Could you check a few things on this model? Use its own coordinates, in mm. Face numbers are marked on the shaded views. A direction names the side the tool comes from. Give positions to 0.01 mm unless a question says otherwise; leave off trailing zeros. Order: outer loops, then holes, each group sorted by start corner. A loop starts at its lowest first (then second) coordinate and runs counter-clockwise, first axis right, second up. Notation, with made-up numbers: M -34.5,12.5 L 5.5,12.5 A32 ccw 5.5,39.5 Z; hole C 3.5,16 d1. An arc over 180 degrees is marked long. Answer in a Markdown table with one row per item. Add a question column.
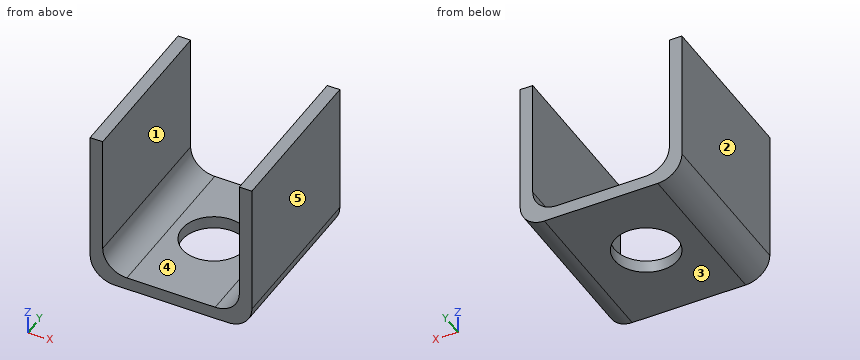
```python
from build123d import *

# Parameters (mm, degrees)
BOSS_EXTRUDE1_DEPTH = 8.636
HOLE1_D             = 3.3274


with BuildPart() as part:
    # Sketch1 → Boss-Extrude1 (new body)
    with BuildSketch(Plane(origin=(0, 11.385459202, 0), x_dir=(-1, 0, 0), z_dir=(0, 1, 0))):
        with BuildLine():
            Line((5.749291724, 0), (11.718291724, 0))
            ThreePointArc((11.718291724, 0), (12.616317336, 0.371974388), (12.988291724, 1.27))
            Line((12.988291724, 1.27), (12.988291724, 8.2296))
            Line((12.988291724, 8.2296), (12.327891724, 8.2296))
            Line((12.327891724, 8.2296), (12.327891724, 1.9304))
            ThreePointArc((12.327891724, 1.9304), (11.955917336, 1.032374388), (11.057891724, 0.6604))
            Line((11.057891724, 0.6604), (6.409691724, 0.6604))
            ThreePointArc((6.409691724, 0.6604), (5.511666112, 1.032374388), (5.139691724, 1.9304))
            Line((5.139691724, 1.9304), (5.139691724, 8.2296))
            Line((5.139691724, 8.2296), (4.479291724, 8.2296))
            Line((4.479291724, 8.2296), (4.479291724, 1.27))
            ThreePointArc((4.479291724, 1.27), (4.851266112, 0.371974388), (5.749291724, 0))
        make_face()
    extrude(amount=-BOSS_EXTRUDE1_DEPTH)

    # Hole1 (through all)
    with Locations(Plane.XY.offset(0.6604)):
        with Locations((-8.886505488, 7.234194178)):
            Hole(HOLE1_D / 2)


solid = part.part
```
1. Suppose I cut it at D-D on x = -6. List the corners of the cut face in (y, z) for me, plus the area to 3 significant figures.
2. Will this pin go through, and if not, where does the flat tip stop? P1, Ø2.5, axis at x = -9, y = 5, coming from the +Z side.
3. If I drill on line 1 along X through (y, z) = (10.75, 2); line 2 along Z through (x, y) = (-10.5, 10); line 3 along X through (y, z) = (5.75, 1.75), over which ranges is the centre line in solid material (lowest first)? Write a range as [from, to].
4. Suppose I cut it at B-B on y = 4. List the corners of the cut face in (x, z) for me.
5. Thinking about a two-plate mould opening in X: for the marked faces 3, 4 and 5, which applies, pulls with the +X half, pulls with the -X half, needs draft (parallel to the pull), parting line crosses it, or undercut?
6. Suppose I cut it at A-A on z = 4.75. List the corners of the cut face in (x, y) for me.
7. Suppose I cut it at C-C on y = 8. List the corners of the cut face in (x, z) for me, plus the area to 3 significant figures.
8. For the marked faces 1 and 2, which set-ups out of +Z, -Z, +X, -X, +Y, -Y let a thin tool reach every point of the face, with its end or its side?
Findings below:
| question | item | result |
|---|---|---|
| 1 | outline | M 2.75,0 L 11.39,0 L 11.39,0.73 L 2.75,0.73 Z |
| 1 | area | 6.29 mm2 |
| 2 | P1 | z = 0.66 |
| 3 | line 1 | [-12.99, -12.33], [-5.14, -4.48] |
| 3 | line 2 | [0, 0.66] |
| 3 | line 3 | [-12.99, -12.32], [-5.15, -4.48] |
| 4 | outline | M -12.99,1.27 A1.27 ccw -11.72,0 L -5.75,0 A1.27 ccw -4.48,1.27 L -4.48,8.23 L -5.14,8.23 L -5.14,1.93 A1.27 cw -6.41,0.66 L -11.06,0.66 A1.27 cw -12.33,1.93 L -12.33,8.23 L -12.99,8.23 Z |
| 5 | face 3 | needs draft |
| 5 | face 4 | undercut |
| 5 | face 5 | pulls with the +X half |
| 6 | outline | M -12.99,2.75 L -12.33,2.75 L -12.33,11.39 L -12.99,11.39 Z; M -5.14,2.75 L -4.48,2.75 L -4.48,11.39 L -5.14,11.39 Z |
| 7 | outline | M -12.99,1.27 A1.27 ccw -11.72,0 L -10.36,0 L -10.36,0.66 L -11.06,0.66 A1.27 cw -12.33,1.93 L -12.33,8.23 L -12.99,8.23 Z; M -7.41,0 L -5.75,0 A1.27 ccw -4.48,1.27 L -4.48,8.23 L -5.14,8.23 L -5.14,1.93 A1.27 cw -6.41,0.66 L -7.41,0.66 Z |
| 7 | area | 13.7 mm2 |
| 8 | face 1 | +Z, +Y, -Y |
| 8 | face 2 | +Z, -Z, -X, +Y, -Y |
